Part model, mm, in its own coordinate system. Give positions to 0.01 mm unless a question says otherwise; leave off trailing zeros. Write each loop counter-clockwise with the first axis right and the second up, starting at its lowest first coordinate (ties: lowest second). Pieces come first, ordered by that corner, then holes.
```python
from build123d import *

# Parameters (mm, degrees)
F1_DEPTH = 377.5
F2_R     = 5
F3_R     = 5
F5_D     = 4.2
F7_D     = 2.5


with BuildPart() as f1:
    # F0 (on Front) → F1 (new body)
    with BuildSketch(Plane.XZ):
        Polygon((0, 15), (0, 0), (30, 0), (30, 15), (27, 15), (27, 3.5), (3, 3.5), (3, 15), align=None)
    extrude(amount=F1_DEPTH)

    # F2
    f2_edges = [f1.edges().sort_by_distance(p)[0] for p in [
        (3, -188.75, 3.5),
    ]]
    fillet(f2_edges, radius=F2_R)

    # F3
    f3_edges = [f1.edges().sort_by_distance(p)[0] for p in [
        (27, -188.75, 3.5),
    ]]
    fillet(f3_edges, radius=F3_R)

    # F5 (through all)
    with Locations(Plane(origin=(0, 0, 0), x_dir=(1, 0, 0), z_dir=(0, 0, -1))):
        with Locations((24, 32), (15, 16), (6, 32)):
            Hole(F5_D / 2)

    # F7 (through all)
    with Locations(Plane(origin=(0, 0, 0), x_dir=(1, 0, 0), z_dir=(0, 0, -1))):
        with Locations((20.5, 151), (20.5, 141), (20.5, 131), (15, 146), (15, 136), (9.5, 151), (9.5, 141), (9.5, 131), (20.5, 215), (20.5, 205), (20.5, 195), (15, 210), (15, 200), (9.5, 215), (9.5, 205), (9.5, 195)):
            Hole(F7_D / 2)

    # F8: F1 across face


with BuildPart() as f1_1:
    add(f1.part)
    add(f1.part.mirror(Plane(origin=(15, -377.5, 4.7179054872), x_dir=(1, 0, 0), z_dir=(0, -1, 0))))


solid = f1_1.part
```
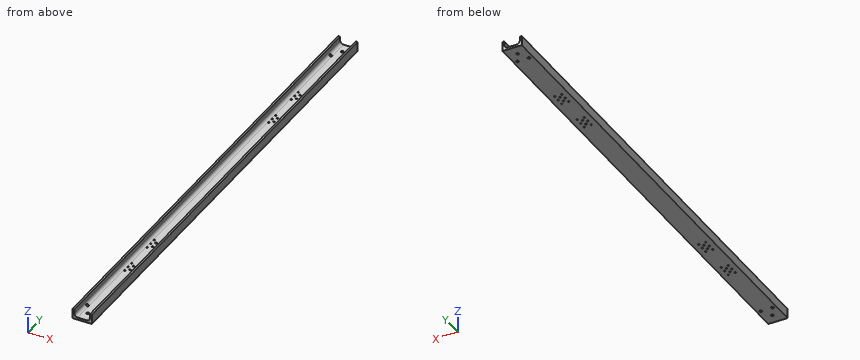
1) Saw through at B-B, the plane y = -247.5. Write the cut outline in (x, z).
Answers follow:
outline: (0, 0) - (30, 0) - (30, 15) - (27, 15) - (27, 8.5) arc R5 cw to (22, 3.5) - (8, 3.5) arc R5 cw to (3, 8.5) - (3, 15) - (0, 15) - close
2) Pin check, flat tip, straight feed: pin 1 Ø3 at (x, y) = (15, -609) entering from +Z. Stop position of the tip, or through.
Answers follow:
pin 1: stops at z = 3.5
3) Saw through at A-A, the plane z = 12.5. Write the cut outline in (x, y).
Answers follow:
outline: (0, -755) - (3, -755) - (3, 0) - (0, 0) - close; (27, -755) - (30, -755) - (30, 0) - (27, 0) - close
4) Wall check: L1, parallel to Y at x = 6, z = 2.7; L2, parallel to X at y = -228, z = 8.75; L3, parallel to X at y = -141, z = 2.35. Give the ranges that are in metal, low to high.
Answers follow:
L1: y = -755 to -725.1, -720.9 to -34.1, -29.9 to 0
L2: x = 0 to 3, 27 to 30
L3: x = 0 to 8.25, 10.75 to 19.25, 21.75 to 30
